Verification items for the finished model (mm, model axes). A direction names the side the tool comes from. Coordinates: 2 decimals unless noted, no trailing zeros. Write each loop counter-clockwise with the first axis right and the second up, starting at its lowest first coordinate (ties: lowest second). Pieces come first, ordered by that corner, then holes. Notation, with made-up numbers: M 79.25,-34 L 108.25,-34 A24 ccw 108.25,-10 Z; hole C -25.75,38 d11. An arc over 180 degrees is marked long. Answer in a Markdown table with one row per item.
from build123d import *

# Parameters (mm, degrees)
BOSS_EXTRU_2_DEPTH                            = 1
ESQUISSE4_R                                   = 3
BOSS_EXTRU_5_DEPTH                            = 1
TROU_POUR_TARAUDAGE_POUR_TROU_TARAUD_M2_D     = 1.6
TROU_POUR_TARAUDAGE_POUR_TROU_TARAUD_M2_DEPTH = 10
TROU_POUR_TARAUDAGE_POUR_TROU_TARAUD_M2_TIP   = 0.480688495
ESQUISSE8_R                                   = 13.8
BOSS_EXTRU_6_DEPTH                            = 11
CHANFREIN1_SIZE                               = 3
ESQUISSE13_R                                  = 4
BOSS_EXTRU_7_DEPTH                            = 4.35
ESQUISSE14_R                                  = 1.583459573
BOSS_EXTRU_8_DEPTH                            = 1.5


with BuildPart() as part:
    # Esquisse3 → Boss.-Extru.2 (new body)
    with BuildSketch(Plane.XY):
        Polygon((-44.638743765, 23.961876808), (-44.638743765, 11.211876808), (-57.388743765, 11.211876808), (-57.388743765, 5.211876808), (-44.638743765, 5.211876808), (-44.638743765, -7.538123192), (-38.638743765, -7.538123192), (-38.638743765, 5.211876808), (-25.888743765, 5.211876808), (-25.888743765, 11.211876808), (-38.638743765, 11.211876808), (-38.638743765, 23.961876808), align=None)
    extrude(amount=BOSS_EXTRU_2_DEPTH)

    # Esquisse4 → Boss.-Extru.5 (add)
    with BuildSketch(Plane.XY.offset(1)):
        with Locations((-41.638743765, 23.961876808)):
            Circle(ESQUISSE4_R)
        with Locations((-25.888743765, 8.211876808)):
            Circle(ESQUISSE4_R)
        with Locations((-41.638743765, -7.538123192)):
            Circle(ESQUISSE4_R)
        with Locations((-57.388743765, 8.211876808)):
            Circle(ESQUISSE4_R)
    extrude(amount=-BOSS_EXTRU_5_DEPTH)

    # Trou pour taraudage pour trou taraudé M2x0.41
    with Locations(Plane.XY.offset(1)):
        with Locations((-41.638743765, 24.561876808), (-25.288743765, 8.211876808), (-41.638743765, -8.138123192), (-57.988743765, 8.211876808)):
            Hole(TROU_POUR_TARAUDAGE_POUR_TROU_TARAUD_M2_D / 2, depth=TROU_POUR_TARAUDAGE_POUR_TROU_TARAUD_M2_DEPTH)
            with Locations((0, 0, -(TROU_POUR_TARAUDAGE_POUR_TROU_TARAUD_M2_DEPTH + TROU_POUR_TARAUDAGE_POUR_TROU_TARAUD_M2_TIP / 2))):  # 118° drill point
                Cone(0, TROU_POUR_TARAUDAGE_POUR_TROU_TARAUD_M2_D / 2, TROU_POUR_TARAUDAGE_POUR_TROU_TARAUD_M2_TIP, mode=Mode.SUBTRACT)

    # Esquisse8 → Boss.-Extru.6 (add)
    with BuildSketch(Plane.XY.offset(1)):
        with Locations((-41.638743765, 8.211876808)):
            Circle(ESQUISSE8_R)
    extrude(amount=BOSS_EXTRU_6_DEPTH)

    # Chanfrein1
    chanfrein1_edges = [part.edges().sort_by_distance(p)[0] for p in [
        (-55.438743765, 8.211876808, 12),
    ]]
    chamfer(chanfrein1_edges, length=CHANFREIN1_SIZE)

    # Esquisse13 → Boss.-Extru.7 (add)
    with BuildSketch(Plane.XY.offset(12)):
        with Locations((-41.638743765, 8.211876808)):
            Circle(ESQUISSE13_R)
    extrude(amount=BOSS_EXTRU_7_DEPTH)

    # Esquisse14 → Boss.-Extru.8 (add)
    with BuildSketch(Plane.XY.offset(16.35)):
        with Locations((-41.638743765, 8.211876808)):
            Circle(ESQUISSE14_R)
    extrude(amount=BOSS_EXTRU_8_DEPTH)


solid = part.part
1) Sectioned sample at B-B (z = 11.5). Record the cut outline in (x, y).
Response values:
| item | result |
|---|---|
| outline | C -41.64,8.21 d22.6 |
2) Tool access check on faces 1 (the face through (-44.639, 17.7, 0.5)), 2 (the face through (-38.639, -1.3, 0.5)), 3 (the face through (-42, 6, 16.35)), 4 (the face through (-38.639, 17.5, 0.5)). Record the directions out of +Z, -Z, +X, -X, +Y, -Y that give a thin tool (end or side, any length) a straight path to the whole face; none if there is none.
Response values:
| item | result |
|---|---|
| face 1 | -Z, -X, +Y |
| face 2 | -Z, +X, -Y |
| face 3 | +Z |
| face 4 | -Z, +X, +Y |
3) Sectioned sample at A-A (y = -6.5). Record the cut outline in (x, z), then the cut area to 3 significant figures.
Response values:
| item | result |
|---|---|
| outline | M -44.64,0 L -38.64,0 L -38.64,1 L -44.64,1 Z |
| area | 6.00 mm² |
4) Depth check by flat-ended pin: pin 1 (1.6 mm diameter, centred on x = -59, y = 7, fed in from +Z); pin 2 (8.5 mm diameter, centred on x = -48, y = 1, fed in from -Z); pin 3 (2 mm diameter, centred on x = -51, z = 5.5, fed in from +Y); pin 4 (3 mm diameter, centred on x = -52, z = 6.5, fed in from -Y). Enter the tip coordinate at first touch or a pass-through.
Response values:
| item | result |
|---|---|
| pin 1 | stops at z = 1 |
| pin 2 | stops at z = 0 |
| pin 3 | stops at y = 19.19 |
| pin 4 | stops at y = -2.37 |
5) Sectioned sample at C-C (z = 5.5). Record the cut outline in (x, y).
Response values:
| item | result |
|---|---|
| outline | C -41.64,8.21 d27.6 |
6) Thickness scan on L1, parallel to Y at x = -39, z = 14; L2, parallel to Z at x = -56.5, y = 6; L3, parallel to Z at x = -37.5, y = 6. Record the ranges inside material, lowest first. Write a range as [from, to].
Response values:
| item | result |
|---|---|
| L1 | y = [5.21, 11.22] |
| L2 | z = [0, 1] |
| L3 | z = [0, 12] |
